```python
from build123d import *

# Parameters (mm, degrees)
F0_R     = 25.4
F0_R_2   = 1.5
F1_DEPTH = 5.08


with BuildPart() as f1:
    # F0 (on Top) → F1 (new body)
    with BuildSketch(Plane.XY):
        with BuildLine():
            ThreePointArc((355.6, 83.9), (354.135534, 87.435534), (350.6, 88.9))
            Line((350.6, 88.9), (-350.6, 88.9))
            ThreePointArc((-350.6, 88.9), (-354.135534, 87.435534), (-355.6, 83.9))
            Line((-355.6, 83.9), (-355.6, -83.9))
            ThreePointArc((-355.6, -83.9), (-354.135534, -87.435534), (-350.6, -88.9))
            Line((-350.6, -88.9), (350.6, -88.9))
            ThreePointArc((350.6, -88.9), (354.135534, -87.435534), (355.6, -83.9))
            Line((355.6, -83.9), (355.6, 83.9))
        make_face()
        with BuildLine():
            ThreePointArc((-333.7, -53.3), (-335.2, -54.8), (-336.7, -53.3))
            Line((-336.7, -53.3), (-336.7, -48.3))
            ThreePointArc((-336.7, -48.3), (-335.2, -46.8), (-333.7, -48.3))
            Line((-333.7, -48.3), (-333.7, -53.3))
        make_face(mode=Mode.SUBTRACT)
        with BuildLine():
            ThreePointArc((-15.53033, -16.59099), (-16.59099, -16.59099), (-16.59099, -15.53033))
            Line((-16.59099, -15.53033), (-14.46967, -13.40901))
            ThreePointArc((-14.46967, -13.40901), (-13.40901, -13.40901), (-13.40901, -14.46967))
            Line((-13.40901, -14.46967), (-15.53033, -16.59099))
        make_face(mode=Mode.SUBTRACT)
        with BuildLine():
            Line((333.7, -53.3), (333.7, -48.3))
            ThreePointArc((333.7, -48.3), (335.2, -46.8), (336.7, -48.3))
            Line((336.7, -48.3), (336.7, -53.3))
            ThreePointArc((336.7, -53.3), (335.2, -54.8), (333.7, -53.3))
        make_face(mode=Mode.SUBTRACT)
        with BuildLine():
            ThreePointArc((16.59099, -15.53033), (16.59099, -16.59099), (15.53033, -16.59099))
            Line((15.53033, -16.59099), (13.40901, -14.46967))
            ThreePointArc((13.40901, -14.46967), (13.40901, -13.40901), (14.46967, -13.40901))
            Line((14.46967, -13.40901), (16.59099, -15.53033))
        make_face(mode=Mode.SUBTRACT)
        with Locations((-295.2, 0)):
            Circle(F0_R, mode=Mode.SUBTRACT)
        with BuildLine():
            ThreePointArc((-13.40901, 14.46967), (-13.40901, 13.40901), (-14.46967, 13.40901))
            Line((-14.46967, 13.40901), (-16.59099, 15.53033))
            ThreePointArc((-16.59099, 15.53033), (-16.59099, 16.59099), (-15.53033, 16.59099))
            Line((-15.53033, 16.59099), (-13.40901, 14.46967))
        make_face(mode=Mode.SUBTRACT)
        with Locations((-19.05, 38.1)):
            Circle(F0_R_2, mode=Mode.SUBTRACT)
        with Locations((-335.2, 50.8)):
            Circle(F0_R_2, mode=Mode.SUBTRACT)
        with Locations((-19.05, 76.2)):
            Circle(F0_R_2, mode=Mode.SUBTRACT)
        with BuildLine():
            ThreePointArc((14.46967, 13.40901), (13.40901, 13.40901), (13.40901, 14.46967))
            Line((13.40901, 14.46967), (15.53033, 16.59099))
            ThreePointArc((15.53033, 16.59099), (16.59099, 16.59099), (16.59099, 15.53033))
            Line((16.59099, 15.53033), (14.46967, 13.40901))
        make_face(mode=Mode.SUBTRACT)
        with Locations((19.05, 38.1)):
            Circle(F0_R_2, mode=Mode.SUBTRACT)
        with Locations((295.2, 0)):
            Circle(F0_R, mode=Mode.SUBTRACT)
        with Locations((19.05, 76.2)):
            Circle(F0_R_2, mode=Mode.SUBTRACT)
        with Locations((335.2, 50.8)):
            Circle(F0_R_2, mode=Mode.SUBTRACT)
    extrude(amount=F1_DEPTH)


solid = f1.part
```
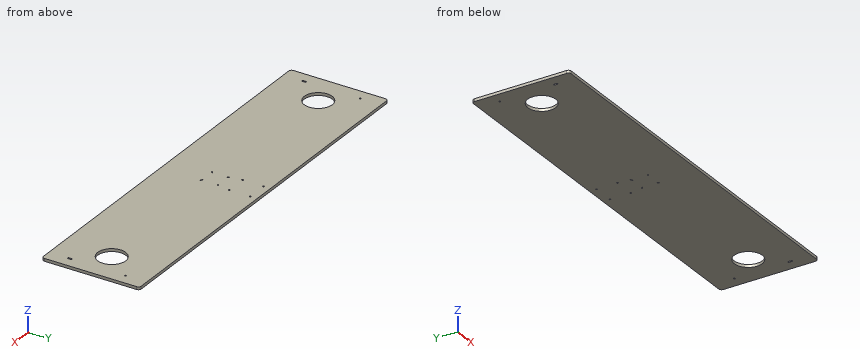
Here's how the part is built. I have some questions about the finished solid (model axes, mm). Coordinates: 2 decimals unless noted, no trailing zeros. Loops run counter-clockwise (first coordinate to the right, second up) from the corner with the lowest first, then second, coordinate; pieces in that order, holes last. Notation, with made-up numbers: M -13.75,60 L -7.75,60 A23 cw -7.75,68 Z; hole C -32,62 d9. An arc over 180 degrees is marked long. One line per item, written item: value.
1. Imagine slicing it at C-C (z = 1.9). State how many separate pieces and enclosed holes the cut face has, and give its area (3 significant figures).
Geometry says:
separate pieces: 1
enclosed holes: 14
area: 122,000 mm2
2. Imagine slicing it at D-D (x = -298). List the corners of the cut face in (y, z) for me.
Geometry says:
outline: M -88.9,0 L -25.25,0 L -25.25,5.08 L -88.9,5.08 Z; M 25.25,0 L 88.9,0 L 88.9,5.08 L 25.25,5.08 Z
3. Imagine slicing it at B-B (y = 0). List the corners of the cut face in (x, z) for me.
Geometry says:
outline: M -355.6,0 L -320.6,0 L -320.6,5.08 L -355.6,5.08 Z; M -269.8,0 L 269.8,0 L 269.8,5.08 L -269.8,5.08 Z; M 320.6,0 L 355.6,0 L 355.6,5.08 L 320.6,5.08 Z
4. Imagine slicing it at A-A (x = 295.2). List the corners of the cut face in (y, z) for me, and give its area (3 significant figures).
Geometry says:
outline: M -88.9,0 L -25.4,0 L -25.4,5.08 L -88.9,5.08 Z; M 25.4,0 L 88.9,0 L 88.9,5.08 L 25.4,5.08 Z
area: 645 mm2
5. Will this pin go through, and if not, where does the flat tip stop? pin 1 Ø1.8 at (x, y) = (-19.05, 38.1) entering from +Z.
Geometry says:
pin 1: passes through
6. Please list where these lines run through material, in increasing order: probe 1 along Y at (x, z) = (19.05, 2.2); probe 2 along Y at (x, z) = (-335.2, 1.55); probe 3 along X at (y, z) = (76.2, 1.35).
Geometry says:
probe 1: y = -88.9 to 36.6, 39.6 to 74.7, 77.7 to 88.9
probe 2: y = -88.9 to -54.8, -46.8 to 49.3, 52.3 to 88.9
probe 3: x = -355.6 to -20.55, -17.55 to 17.55, 20.55 to 355.6
